The listing builds one solid part. Answer for the finished solid, in the listing's coordinates (mm). Round coordinates to 2 decimals unless told otherwise and drop trailing zeros. Order: outer loops, then holes, each group sorted by start corner. A loop starts at its lowest first (then second) coordinate and runs counter-clockwise, first axis right, second up. Notation, with made-up numbers: (89.5, 80.5) - (120.5, 80.5) arc R26 cw to (120.5, 98.5) - close; hole circle Ø7 at (19, 1.25). An arc over 180 degrees is marked (long way). One line per item, written item: value. Start each with the question number.
1. Section B-B, the plane z = 37 is taken. Count the separate pieces of the cut face and the enclosed holes in it, then the cut area to 4 significant figures.
2. Flat-ended cylindrical pins translate along their axes: P1, Ø6, axis at x = 22.5, y = 210, coming from the +Z side; P2, Ø9.5, axis at x = 6, y = 176.5, coming from the +Z side. Find the tip coordinate at first contact, or state that the pin passes through.
3. For a pull along Y with two mould halves and no side action, classify faces 1 (the flat face through (36.25, 212, -1)), 2 (the flat face through (0, 264.5, 3)) as released by +Y, released by -Y, zero draft, split by the parting line, or undercut.
4. Section A-A, the plane y = 222.5 is taken. Give the vertices of the cut face in (x, z) (3 decimals).
5. Straight lines are drawn through the part: line 1 (X direction, y = 176, z = 24) (3 decimals); line 2 (Z direction, x = 27.5, y = 186.5). For each, find the intervals that lie inside material, in ascending order.
from build123d import *

# Parameters (mm, degrees)
SKETCH1_W           = 72.5
SKETCH1_H           = 95
BOSS_EXTRUDE1_DEPTH = 104.5
SKETCH2_W           = 68.25
SKETCH2_H           = 22.5
CUT_EXTRUDE1_DEPTH  = 90
SKETCH3_W           = 72.5
SKETCH3_H           = 95
BOSS_EXTRUDE2_DEPTH = 175.5
SKETCH4_W           = 68.25
SKETCH4_H           = 12
CUT_EXTRUDE3_DEPTH  = 90
SPLIT1_OUTLINE_W    = 72.5
SPLIT1_OUTLINE_H    = 95
SPLIT1_DEPTH        = 144.5
SKETCH5_W           = 72.5
SKETCH5_H           = 95
BOSS_EXTRUDE3_DEPTH = 2.5


# Read off the part's stored shape, not the designer's step: Split1
with BuildPart() as part:
    # Sketch1 → Boss-Extrude1 (new body)
    with BuildSketch(Plane(origin=(0, 0, 0), x_dir=(1, 0, 0), z_dir=(0, 1, 0))):
        Rectangle(SKETCH1_W, SKETCH1_H)
    extrude(amount=BOSS_EXTRUDE1_DEPTH)

    # Sketch2 → Cut-Extrude1 (cut)
    with BuildSketch(Plane.XY.offset(47.5)):
        with Locations((0, 13.75)):
            Rectangle(SKETCH2_W, SKETCH2_H)
        with Locations((0, 39.25)):
            Rectangle(SKETCH2_W, SKETCH2_H)
        with Locations((0, 64.75)):
            Rectangle(SKETCH2_W, SKETCH2_H)
        with Locations((0, 90.25)):
            Rectangle(SKETCH2_W, SKETCH2_H)
    extrude(amount=-CUT_EXTRUDE1_DEPTH, mode=Mode.SUBTRACT)

    # Sketch3 → Boss-Extrude2 (add)
    with BuildSketch(Plane(origin=(0, 104.5, 0), x_dir=(1, 0, 0), z_dir=(0, 1, 0))):
        Rectangle(SKETCH3_W, SKETCH3_H)
    extrude(amount=BOSS_EXTRUDE2_DEPTH)

    # Sketch4 → Cut-Extrude3 (cut)
    with BuildSketch(Plane.XY.offset(47.5)):
        with Locations((0, 110)):
            Rectangle(SKETCH4_W, SKETCH4_H)
        with Locations((0, 123.5)):
            Rectangle(SKETCH4_W, SKETCH4_H)
        with Locations((0, 137)):
            Rectangle(SKETCH4_W, SKETCH4_H)
        with Locations((0, 150.5)):
            Rectangle(SKETCH4_W, SKETCH4_H)
        with Locations((0, 164)):
            Rectangle(SKETCH4_W, SKETCH4_H)
        with Locations((0, 177.5)):
            Rectangle(SKETCH4_W, SKETCH4_H)
        with Locations((0, 191)):
            Rectangle(SKETCH4_W, SKETCH4_H)
        with Locations((0, 204.5)):
            Rectangle(SKETCH4_W, SKETCH4_H)
        with Locations((0, 218)):
            Rectangle(SKETCH4_W, SKETCH4_H)
        with Locations((0, 231.5)):
            Rectangle(SKETCH4_W, SKETCH4_H)
        with Locations((0, 245)):
            Rectangle(SKETCH4_W, SKETCH4_H)
        with Locations((0, 258.5)):
            Rectangle(SKETCH4_W, SKETCH4_H)
        with Locations((0, 272)):
            Rectangle(SKETCH4_W, SKETCH4_H)
    extrude(amount=-CUT_EXTRUDE3_DEPTH, mode=Mode.SUBTRACT)

    # Split1 outline → Split1 (cut)
    with BuildSketch(Plane(origin=(0, 0, 0), x_dir=(1, 0, 0), z_dir=(0, 1, 0))):
        Rectangle(SPLIT1_OUTLINE_W, SPLIT1_OUTLINE_H)
    extrude(amount=SPLIT1_DEPTH, mode=Mode.SUBTRACT)

    # Sketch5 → Boss-Extrude3 (add)
    with BuildSketch(Plane.XZ.offset(-144.5)):
        Rectangle(SKETCH5_W, SKETCH5_H)
    extrude(amount=BOSS_EXTRUDE3_DEPTH)


solid = part.part
Answer list:
1. separate pieces: 1
1. enclosed holes: 10
1. area: 1,815 mm²
2. P1: stops at z = 47.5
2. P2: stops at z = -42.5
3. face 1: zero draft
3. face 2: undercut
4. outline: (-36.25, -47.5) - (36.25, -47.5) - (36.25, 47.5) - (34.125, 47.5) - (34.125, -42.5) - (-34.125, -42.5) - (-34.125, 47.5) - (-36.25, 47.5) - close
5. line 1: x = -36.25 to -34.125, 34.125 to 36.25
5. line 2: z = -47.5 to -42.5
